Answer from the drawing. Dimensions are ordinates in mm from the lowest x, y and z of the part. Give positions to 0.01 mm unless a question says otherwise; leave off trailing zeros. Loops run counter-clockwise (first coordinate to the right, second up) from the corner with the lowest first, then second, coordinate; pieces in that order, holes last.
(1) Determine the mould class of the marked faces 1, 2, 3 and 4 for opening direction X: pulls with the +X half, pulls with the -X half, needs draft (parallel to the pull), parting line crosses it, or undercut.
(2) Straight lines are drawn through the part: probe 1 along X at (y, z) = (5, 3); probe 2 along X at (y, z) = (4, 14); probe 3 along Y at (x, z) = (29, 4). For each, find the intervals that lie inside material, in ascending order.
(3) Each of these flat-tipped pins is pushed along its axis until it touches: P1, Ø6, axis at y = 17, z = 11, coming from the +X side; P2, Ø1, axis at x = 31.5, z = 32, coming from the +Y side; P3, Ø3.5, axis at x = 47, z = 26.5, coming from the +Y side. Where does it stop, or does it pass through?
(4) Find section B-B, the plane x = 15.5. Write down the section's boundary in (y, z).
(5) Find section C-C, the plane y = 7.5. Write down the section's boundary in (x, z).
(6) Find section A-A, the plane z = 14. Write down the section's boundary in (x, y).
(7) Find section D-D, the plane y = 39. Write down the section's boundary in (x, z).
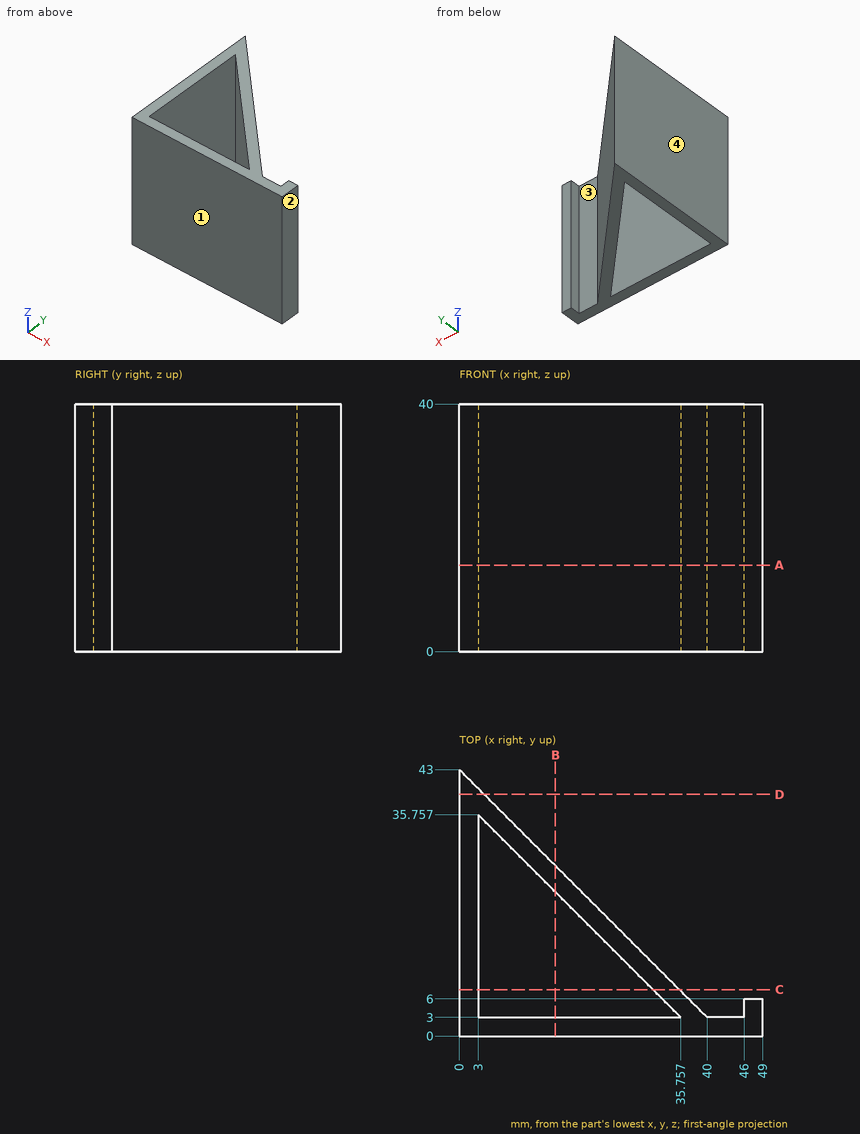
Entries:
1. face 1: needs draft
1. face 2: pulls with the +X half
1. face 3: undercut
1. face 4: pulls with the -X half
2. probe 1: x = 0 to 3, 33.76 to 38, 46 to 49
2. probe 2: x = 0 to 3, 34.76 to 39, 46 to 49
2. probe 3: y = 0 to 3, 9.76 to 14
3. P1: stops at x = 29
3. P2: stops at y = 12
3. P3: stops at y = 6
4. outline: (0, 0) - (3, 0) - (3, 40) - (0, 40) - close; (23.26, 0) - (27.5, 0) - (27.5, 40) - (23.26, 40) - close
5. outline: (0, 0) - (3, 0) - (3, 40) - (0, 40) - close; (31.26, 0) - (35.5, 0) - (35.5, 40) - (31.26, 40) - close
6. outline: (0, 0) - (49, 0) - (49, 6) - (46, 6) - (46, 3) - (40, 3) - (0, 43) - close; hole (3, 3) - (35.76, 3) - (3, 35.76) - close
7. outline: (0, 0) - (4, 0) - (4, 40) - (0, 40) - close
